Geometry check sheet. Reference: the model listing, model coordinates, mm. A direction names the side the tool comes from. Give positions to 0.01 mm unless a question says otherwise; leave off trailing zeros. Loops run counter-clockwise (first coordinate to the right, second up) from the corner with the lowest first, then second, coordinate; pieces in that order, holes last. Notation, with made-up numbers: (23, 3.5) -> (59, 3.5) arc R23 ccw to (59, 24.5) -> close; hole circle Ø4 at (66, 0.25). An arc over 180 degrees is marked (long way). Write item = value, one per line.
```python
from build123d import *

# Parameters (mm, degrees)
PAD002_DEPTH = 5
SKETCH006_R  = 4
PAD003_DEPTH = 5
PAD009_DEPTH = 20


with BuildPart() as part:
    # Sketch003 → Pad002 (new body)
    with BuildSketch(Plane.XY):
        with BuildLine():
            ThreePointArc((0, -45), (45, 0), (0, 45))
            Line((0, 45), (0, 55))
            ThreePointArc((12.5, 53.560713), (6.291295, 54.638994), (0, 55))
            Line((12.5, 50.415026), (12.5, 53.560713))
            ThreePointArc((12.5, 50.415026), (15, 47.915026), (17.5, 50.415026))
            Line((17.5, 50.415026), (17.5, 52.141634))
            ThreePointArc((17.5, -52.141634), (55, 0), (17.5, 52.141634))
            Line((17.5, -50.415026), (17.5, -52.141634))
            ThreePointArc((17.5, -50.415026), (15, -47.915026), (12.5, -50.415026))
            Line((12.5, -50.415026), (12.5, -53.560713))
            ThreePointArc((10, -54.083269), (11.253034, -53.836505), (12.5, -53.560713))
            Line((10, -55), (10, -54.083269))
            ThreePointArc((0, -55), (5, -60), (10, -55))
            Line((0, -45), (0, -55))
        make_face()
    extrude(amount=PAD002_DEPTH)

    # Sketch006 (on Face15 of Pad002) → Pad003 (join)
    with BuildSketch(Plane(origin=(0, 0, 0), x_dir=(1, 0, 0), z_dir=(0, 0, -1))):
        with Locations((5, 55)):
            Circle(SKETCH006_R)
    extrude(amount=PAD003_DEPTH)

    # Sketch009 (on Face18 of Pad003) → Pad009 (join)
    with BuildSketch(Plane(origin=(0, 0, -5), x_dir=(1, 0, 0), z_dir=(0, 0, -1))):
        Polygon((2.113249, 55), (3.556624, 52.5), (6.443376, 52.5), (7.886751, 55), (6.443376, 57.5), (3.556624, 57.5), align=None)
    extrude(amount=PAD009_DEPTH)


with BuildPart() as part_1:
    # Body001 placement: moved
    add(part.part.moved(Location((0, 0, 8))))


solid = part_1.part
```
Item 1: Gauge pin test, flat ends, axial feed: pin 1 (2 mm diameter, centred on x = 37.5, y = -28, fed in from -Z); pin 2 (1.4 mm diameter, centred on x = 4.5, z = -5.5, fed in from -Y); pin 3 (1.4 mm diameter, centred on x = 5, z = -3.5, fed in from +Y). Record the tip position at first contact, or that the pin passes through.
Answer:
pin_1 = 8
pin_2 = -57.5
pin_3 = -52.5
Item 2: Section check B-B, the plane z = -7. Record the cut outline in (x, y), plus the area to 3 significant figures.
Answer:
outline = (2.11, -55) -> (3.56, -57.5) -> (6.44, -57.5) -> (7.89, -55) -> (6.44, -52.5) -> (3.56, -52.5) -> close
area = 21.7 mm^2
Item 3: Section check D-D, the plane x = 15. Record the cut outline in (y, z).
Answer:
outline = (-47.92, 8) -> (-42.43, 8) -> (-42.43, 13) -> (-47.92, 13) -> close; (42.43, 8) -> (47.92, 8) -> (47.92, 13) -> (42.43, 13) -> close
Item 4: Thickness scan on L1, parallel to Z at x = 18, y = -44; L2, parallel to X at y = 1.5, z = 9 (3 decimals); L3, parallel to X at y = 32, z = 9.25. Record the ranges inside material, lowest first. Write a range as [from, to].
Answer:
L1 = [8, 13]
L2 = [44.975, 54.98]
L3 = [31.64, 44.73]
Item 5: Section check C-C, the plane y = 0. Record the cut outline in (x, z).
Answer:
outline = (45, 8) -> (55, 8) -> (55, 13) -> (45, 13) -> close
Item 6: Section check A-A, the plane x = 5. Record the cut outline in (y, z).
Answer:
outline = (-60, 8) -> (-59, 8) -> (-59, 3) -> (-57.5, 3) -> (-57.5, -17) -> (-52.5, -17) -> (-52.5, 3) -> (-51, 3) -> (-51, 8) -> (-44.72, 8) -> (-44.72, 13) -> (-60, 13) -> close; (44.72, 8) -> (54.77, 8) -> (54.77, 13) -> (44.72, 13) -> close
Item 7: Draft check along X on faces 1 (the flat face through (5, -57.5, -7)), 2 (the flat face through (0, -50, 10)), 3 (the cylindrical face through (14.945, 47.916, 10.465)), 4 (the cylindrical face through (4.133, -51.095, 5.535)). Enter one of: +X half, -X half, draft (parallel to the pull), parting line (faces both ways), or undercut.
Answer:
face_1 = draft
face_2 = -X half
face_3 = undercut
face_4 = parting line
Item 8: Tool access check on faces 5 (the flat face through (5, -52.5, -7)), 6 (the flat face through (2.845, -56.268, -6.86)), 7 (the flat face through (12.5, -52, 10)), 8 (the flat face through (5, -52, 3)). Record the directions out of +Z, -Z, +X, -X, +Y, -Y that give a thin tool (end or side, any length) a straight path to the whole face; none if there is none.
Answer:
face_5 = -Z, +X, -X, +Y
face_6 = -Z, -X, -Y
face_7 = +Z, -Z, -Y
face_8 = -Z
